Geometry check sheet. Reference: the model listing, model coordinates, mm. A direction names the side the tool comes from. Give positions to 0.01 mm unless a question says otherwise; leave off trailing zeros. Order: outer loops, then holes, each group sorted by start corner. A loop starts at its lowest first (then second) coordinate and runs counter-clockwise, first axis right, second up. Notation, with made-up numbers: M -5,66.5 L 32,66.5 A37 ccw 32,102.5 Z; hole C -1.5,1.5 d5. An arc over 180 degrees is marked long. Answer as a JSON object with one key per item and string values. Group by question number.
from build123d import *

# Parameters (mm, degrees)
F1_DEPTH = 101.6


with BuildPart() as f1:
    # F0 (on Right) → F1 (new body)
    with BuildSketch(Plane.YZ):
        Polygon((-25.4, 0), (0, 0), (0, 50.8), (-12.7, 50.8), (-12.7, 76.2), (0, 76.2), (0, 101.6), (-25.4, 101.6), (-50.8, 76.2), (-76.2, 101.6), (-101.6, 101.6), (-101.6, 76.2), (-88.9, 76.2), (-88.9, 50.8), (-101.6, 50.8), (-101.6, 0), (-76.2, 0), (-76.2, 25.4), (-25.4, 25.4), align=None)
    extrude(amount=-F1_DEPTH)


solid = f1.part
1. Release check for a two-part mould opening along Z. For faces 5 (the flat face through (-50, -95, 76.2)), 6 (the flat face through (-50, -76.2, 13)), 7 (the flat face through (-50, -38, 89)) record: released by +Z, released by -Z, zero draft, split by the parting line, or undercut.
2. Access from +Z, -Z, +X, -X, +Y, -Y to the whole of each face (thin tool, end or side, straight path). Record for faces 1 (the flat face through (-50, -12.7, 63)), 2 (the flat face through (-50.1, -63.3, 88.7)), 3 (the flat face through (-50, -95, 50.8)), 4 (the flat face through (-50, -25.4, 13)).
3. Thickness scan on line 1 along Z through (x, y) = (-89, -6.5); line 2 along Y through (x, z) = (-83, 22.5); line 3 along Y through (x, z) = (-22.5, 73). Record the ranges inside material, lowest first. Write a range as [from, to].
4. Cross-section at A-A (y = -94). Record the cut outline in (x, z), and give its area (3 significant figures).
5. Depth check by flat-ended pin: pin 1 (10 mm diameter, centred on x = -80.5, z = 67, fed in from -Y); pin 2 (8 mm diameter, centred on x = -53.5, y = -54, fed in from +Z); pin 3 (7.5 mm diameter, centred on x = -51.5, z = 18.5, fed in from +Y). Enter the tip coordinate at first touch or a pass-through.
6. Cross-section at C-C (x = -16). Record the cut outline in (y, z).
7. Cross-section at B-B (z = 22). Record the cut outline in (x, y), and give its area (3 significant figures).
8. Cross-section at D-D (y = -45.5). Record the cut outline in (x, z).
Report:
{
 "1": {"face 5": "undercut", "face 6": "zero draft", "face 7": "released by +Z"},
 "2": {"face 1": "+X, -X, +Y", "face 2": "+Z, +X, -X", "face 3": "+X, -X, -Y", "face 4": "-Z, +X, -X"},
 "3": {"line 1": "z = [0, 50.8], [76.2, 101.6]", "line 2": "y = [-101.6, -76.2], [-25.4, 0]", "line 3": "y = [-88.9, -12.7]"},
 "4": {"outline": "M -101.6,0 L 0,0 L 0,50.8 L -101.6,50.8 Z; M -101.6,76.2 L 0,76.2 L 0,101.6 L -101.6,101.6 Z", "area": "7,740 mm2"},
 "5": {"pin 1": "stops at y = -88.9", "pin 2": "stops at z = 83.4", "pin 3": "stops at y = 0"},
 "6": {"outline": "M -101.6,0 L -76.2,0 L -76.2,25.4 L -25.4,25.4 L -25.4,0 L 0,0 L 0,50.8 L -12.7,50.8 L -12.7,76.2 L 0,76.2 L 0,101.6 L -25.4,101.6 L -50.8,76.2 L -76.2,101.6 L -101.6,101.6 L -101.6,76.2 L -88.9,76.2 L -88.9,50.8 L -101.6,50.8 Z"},
 "7": {"outline": "M -101.6,-101.6 L 0,-101.6 L 0,-76.2 L -101.6,-76.2 Z; M -101.6,-25.4 L 0,-25.4 L 0,0 L -101.6,0 Z", "area": "5,160 mm2"},
 "8": {"outline": "M -101.6,25.4 L 0,25.4 L 0,81.5 L -101.6,81.5 Z"}
}
